Verification items for the finished model (mm, model axes). Face numbers are marked on the shaded views. A direction names the side the tool comes from. Give positions to 0.01 mm unless a question says otherwise; leave off trailing zeros. Loops run counter-clockwise (first coordinate to the right, second up) from the corner with the lowest first, then second, coordinate; pieces in that order, holes last. Notation, with made-up numbers: M 77,84.25 L 97,84.25 A15 cw 97,97.25 Z; hole C -23,13 d3. An arc over 180 degrees is marked long. Write each question's results on one line, items separated by ' | '. Start each with the question number.
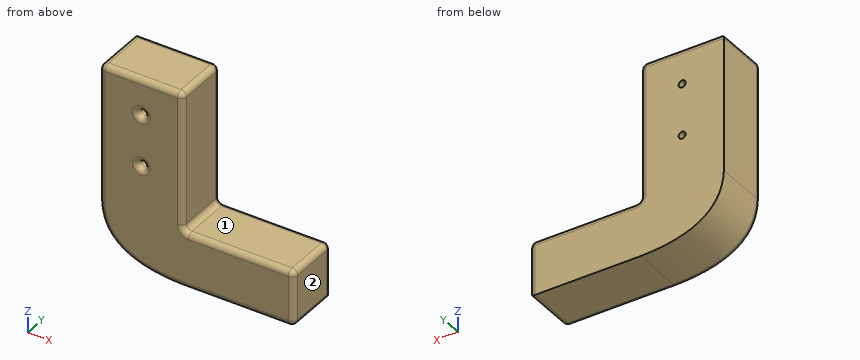
```python
from build123d import *

# Parameters (mm, degrees)
F0_W     = 38.1
F0_H     = 63.5
F0_W_2   = 50.8
F0_H_2   = 25.4
F1_DEPTH = 25.4
F3_D     = 3.2
F4_R     = 2.54


with BuildPart() as f1:
    # F0 (on Front) → F1 (new body)
    with BuildSketch(Plane.XZ):
        with Locations((-19.05, 31.75)):
            Rectangle(F0_W, F0_H)
        with BuildLine():
            Line((0, 0), (-38.1, 0))
            add(Edge.make_bspline(
                [(-38.1, 0), (-37.4712883283, -17.6039609522), (-22.7908427074, -25.0856452655), (0, -25.4)],
                knots=[0, 0, 0, 0, 45.7905011984, 45.7905011984, 45.7905011984, 45.7905011984], degree=3))
            Line((0, -25.4), (0, 0))
        make_face()
        with Locations((25.4, -12.7)):
            Rectangle(F0_W_2, F0_H_2)
    extrude(amount=F1_DEPTH)

    # F3 (through all)
    with Locations(Plane.XZ.offset(25.4)):
        with Locations((-19.0056972206, 47.0490716398), (-19.0056972206, 23.3916286379)):
            Hole(F3_D / 2)

    # F4
    f4_edges = [f1.edges().sort_by_distance(p)[0] for p in [
        (-19.05, -25.4, 63.5),
        (0, -25.4, 31.75),
        (-38.1, -25.4, 31.75),
        (25.4, -25.4, 0),
        (-25.00043, -25.4, -20.504125),
        (50.8, -25.4, -12.7),
        (25.4, -25.4, -25.4),
        (-20.605697, -25.4, 23.391629),
        (-20.605697, -25.4, 47.049072),
        (0, -12.7, 63.5),
        (-38.1, -12.7, 63.5),
        (-19.05, 0, 63.5),
        (0, -12.7, 0),
        (0, 0, 31.75),
        (25.4, 0, 0),
        (50.8, -12.7, -25.4),
        (50.8, -12.7, 0),
        (50.8, 0, -12.7),
    ]]
    fillet(f4_edges, radius=F4_R)


solid = f1.part
```
1. Section check A-A, the plane z = 57. Record the boundary of the cut face in (x, y).
2. Depth check by flat-ended pin: pin 1 Ø6 at (x, y) = (27.5, -13.5) entering from +Z; pin 2 Ø10 at (y, z) = (-10, 28.5) entering from +X; pin 3 Ø5 at (x, z) = (-19.01, 23.39) entering from -Y. Enter the tip coordinate at first touch or a pass-through.
3. Section check C-C, the plane y = -24. State how many separate pieces and enclosed holes the cut face has, plus the area to 3 significant figures.
4. Set-up check for the marked faces 1 and 2: record each of +Z, -Z, +X, -X, +Y, -Y from which the full face is reachable in a straight line by a thin tool's end or side.
5. Section check B-B, the plane x = 17.5. Record the boundary of the cut face in (y, z), plus the area to 3 significant figures.
6. Thickness scan on probe 1 along X at (y, z) = (-7, 36); probe 2 along Z at (x, y) = (41, -6); probe 3 along X at (y, z) = (-12.75, 48.5). Record the ranges inside material, lowest first.
Filled sheet:
1) outline: M -38.1,-22.86 A2.54 ccw -35.56,-25.4 L -2.54,-25.4 A2.54 ccw 0,-22.86 L 0,-2.54 A2.54 ccw -2.54,0 L -38.1,0 Z
2) pin 1: z = 0 | pin 2: x = 0 | pin 3: y = -24.8
3) separate pieces: 1 | enclosed holes: 2 | area: 4,380 mm2
4) face 1: +Z, +X, +Y, -Y | face 2: +Z, -Z, +X, +Y, -Y
5) outline: M -25.4,-22.86 A2.54 ccw -22.86,-25.4 L 0,-25.4 L 0,-2.54 A2.54 ccw -2.54,0 L -22.86,0 A2.54 ccw -25.4,-2.54 Z | area: 641 mm2
6) probe 1: -38.1 to 0 | probe 2: -25.4 to 0 | probe 3: -38.1 to -19.68, -18.33 to 0
